```python
from build123d import *

# Parameters (mm, degrees)
Y_KSEKLIK_EKSTR_ZYON1_DEPTH = 12
Y_KSEKLIK_EKSTR_ZYON2_DEPTH = 6
IZIM1_4_R                   = 19
IZIM1_4_R_2                 = 12
Y_KSEKLIK_EKSTR_ZYON3_DEPTH = 12
IZIM1_5_W                   = 6
IZIM1_5_H                   = 10
Y_KSEKLIK_EKSTR_ZYON4_DEPTH = 6
KES_EKSTR_ZYON1_DEPTH       = 11
F_6_0_6_AP_DELIK1_D         = 6
KES_EKSTR_ZYON2_DEPTH       = 4
RADYUS1_R                   = 1
RADYUS2_R                   = 1
IZIM9_R                     = 1
KES_EKSTR_ZYON3_DEPTH       = 50
IZIM10_R                    = 1
KES_EKSTR_ZYON4_DEPTH       = 16
RADYUS3_R                   = 2


with BuildPart() as part:
    # Çizim1 → Yükseklik-Ekstrüzyon1 (new body, symmetric)
    with BuildSketch(Plane.XY):
        with BuildLine():
            Line((-20, 0), (-15, 0))
            ThreePointArc((-15, 0), (0, 15), (15, 0))
            Line((15, 0), (20, 0))
            ThreePointArc((20, 0), (0, 20), (-20, 0))
        make_face()
    extrude(amount=Y_KSEKLIK_EKSTR_ZYON1_DEPTH, both=True)

    # Çizim1<3> → Yükseklik-Ekstrüzyon2 (add, symmetric)
    with BuildSketch(Plane.XY):
        with BuildLine():
            Line((-10, 82.394505579), (-16.180060624, 11.756089409))
            ThreePointArc((-16.180060624, 11.756089409), (0, 20), (16.180060624, 11.756089409))
            Line((16.180060624, 11.756089409), (10, 82.394505579))
            ThreePointArc((10, 82.394505579), (0, 79.55), (-10, 82.394505579))
        make_face()
    extrude(amount=Y_KSEKLIK_EKSTR_ZYON2_DEPTH, both=True)

    # Çizim1<4> → Yükseklik-Ekstrüzyon3 (add, symmetric)
    with BuildSketch(Plane.XY):
        with Locations((0, 98.55)):
            Circle(IZIM1_4_R)
        with Locations((0, 98.55)):
            Circle(IZIM1_4_R_2, mode=Mode.SUBTRACT)
    extrude(amount=Y_KSEKLIK_EKSTR_ZYON3_DEPTH, both=True)

    # Çizim1<5> → Yükseklik-Ekstrüzyon4 (add, symmetric)
    with BuildSketch(Plane.XY):
        with Locations((-27, 5)):
            Rectangle(IZIM1_5_W, IZIM1_5_H)
        with BuildLine():
            Line((-24, 0), (-20, 0))
            ThreePointArc((-20, 0), (-19.318516526, 5.176380902), (-17.320508076, 10))
            Line((-17.320508076, 10), (-24, 10))
            Line((-24, 10), (-24, 0))
        make_face()
        with BuildLine():
            ThreePointArc((17.320508076, 10), (19.318516526, 5.176380902), (20, 0))
            Line((20, 0), (24, 0))
            Line((24, 0), (24, 10))
            Line((24, 10), (17.320508076, 10))
        make_face()
        with Locations((27, 5)):
            Rectangle(IZIM1_5_W, IZIM1_5_H)
    extrude(amount=Y_KSEKLIK_EKSTR_ZYON4_DEPTH, both=True)

    # Çizim2 → Kes-Ekstrüzyon1 (cut, through all)
    with BuildSketch(Plane(origin=(0, 10, 0), x_dir=(1, 0, 0), z_dir=(0, 1, 0))):
        with BuildLine():
            ThreePointArc((-30, 0), (-28.242640687, 4.242640687), (-24, 6))
            Line((-24, 6), (-30, 6))
            Line((-30, 6), (-30, 0))
        make_face()
        with BuildLine():
            Line((-30, -6), (-24, -6))
            ThreePointArc((-24, -6), (-28.242640687, -4.242640687), (-30, 0))
            Line((-30, 0), (-30, -6))
        make_face()
    kes_ekstr_zyon1 = extrude(amount=-KES_EKSTR_ZYON1_DEPTH, mode=Mode.SUBTRACT)

    # Ø6.0 (6) Çap Delik1 (through all)
    with Locations(Plane(origin=(0, 10, 0), x_dir=(1, 0, 0), z_dir=(0, 1, 0))):
        with Locations((-24, 0)):
            f_6_0_6_ap_delik1 = Hole(F_6_0_6_AP_DELIK1_D / 2)

    # Aynalama1: Ø6.0 (6) Çap Delik1 across plane
    add(f_6_0_6_ap_delik1.mirror(Plane(origin=(0, 0, 0), x_dir=(0, 0, 1), z_dir=(1, 0, 0))), mode=Mode.SUBTRACT)

    # Çizim8 → Kes-Ekstrüzyon2 (cut)
    with BuildSketch(Plane.XY.offset(6)):
        with BuildLine():
            Line((5.845451143, 72.512650075), (9.562487885, 30.026725708))
            ThreePointArc((9.562487885, 30.026725708), (9.044653162, 28.501233808), (7.570098489, 27.852414223))
            Line((7.570098489, 27.852414223), (-7.570098489, 27.852414223))
            ThreePointArc((-7.570098489, 27.852414223), (-9.044653162, 28.501233808), (-9.562487885, 30.026725708))
            Line((-9.562487885, 30.026725708), (-5.845451143, 72.512650075))
            ThreePointArc((-5.845451143, 72.512650075), (-5.204242163, 73.812893263), (-3.853061747, 74.338338589))
            Line((-3.853061747, 74.338338589), (3.853061747, 74.338338589))
            ThreePointArc((3.853061747, 74.338338589), (5.204242163, 73.812893263), (5.845451143, 72.512650075))
        make_face()
    kes_ekstr_zyon2 = extrude(amount=-KES_EKSTR_ZYON2_DEPTH, mode=Mode.SUBTRACT)

    # Aynalama2: Kes-Ekstrüzyon2 across plane
    add(kes_ekstr_zyon2.mirror(Plane.XY), mode=Mode.SUBTRACT)

    # Radyus1
    radyus1_edges = [part.edges().sort_by_distance(p)[0] for p in [
        (5.204242163, 73.812893263, 2),
        (7.703969514, 51.269687892, 2),
        (9.044653162, 28.501233808, 2),
        (0, 27.852414223, 2),
        (-9.044653162, 28.501233808, 2),
        (-7.703969514, 51.269687892, 2),
        (-5.204242163, 73.812893263, 2),
        (0, 74.338338589, 2),
        (5.204242163, 73.812893263, 6),
        (0, 74.338338589, 6),
        (-5.204242163, 73.812893263, 6),
        (-7.703969514, 51.269687892, 6),
        (-9.044653162, 28.501233808, 6),
        (0, 27.852414223, 6),
        (9.044653162, 28.501233808, 6),
        (7.703969514, 51.269687892, 6),
    ]]
    fillet(radyus1_edges, radius=RADYUS1_R)

    # Radyus2
    radyus2_edges = [part.edges().sort_by_distance(p)[0] for p in [
        (5.204242163, 73.812893263, -6),
        (0, 74.338338589, -6),
        (-5.204242163, 73.812893263, -6),
        (-7.703969514, 51.269687892, -6),
        (-9.044653162, 28.501233808, -6),
        (0, 27.852414223, -6),
        (9.044653162, 28.501233808, -6),
        (7.703969514, 51.269687892, -6),
        (5.204242163, 73.812893263, -2),
        (0, 74.338338589, -2),
        (-5.204242163, 73.812893263, -2),
        (-7.703969514, 51.269687892, -2),
        (-9.044653162, 28.501233808, -2),
        (0, 27.852414223, -2),
        (9.044653162, 28.501233808, -2),
        (7.703969514, 51.269687892, -2),
    ]]
    fillet(radyus2_edges, radius=RADYUS2_R)

    # Aynalama3: Kes-Ekstrüzyon1 across plane
    add(kes_ekstr_zyon1.mirror(Plane(origin=(0, 0, 0), x_dir=(0, 0, 1), z_dir=(1, 0, 0))), mode=Mode.SUBTRACT)

    # Çizim9 → Kes-Ekstrüzyon3 (cut, through all)
    with BuildSketch(Plane(origin=(19, 0, 0), x_dir=(0, 0, -1), z_dir=(1, 0, 0))):
        with Locations((0, 98.55)):
            Circle(IZIM9_R)
    extrude(amount=-KES_EKSTR_ZYON3_DEPTH, mode=Mode.SUBTRACT)

    # Çizim10 → Kes-Ekstrüzyon4 (cut)
    with BuildSketch(Plane(origin=(0, 117.55, 0), x_dir=(1, 0, 0), z_dir=(0, 1, 0))):
        Circle(IZIM10_R)
    extrude(amount=-KES_EKSTR_ZYON4_DEPTH, mode=Mode.SUBTRACT)

    # Radyus3
    radyus3_edges = [part.edges().sort_by_distance(p)[0] for p in [
        (10, 82.394505579, 0),
        (-10, 82.394505579, 0),
    ]]
    fillet(radyus3_edges, radius=RADYUS3_R)


solid = part.part
```
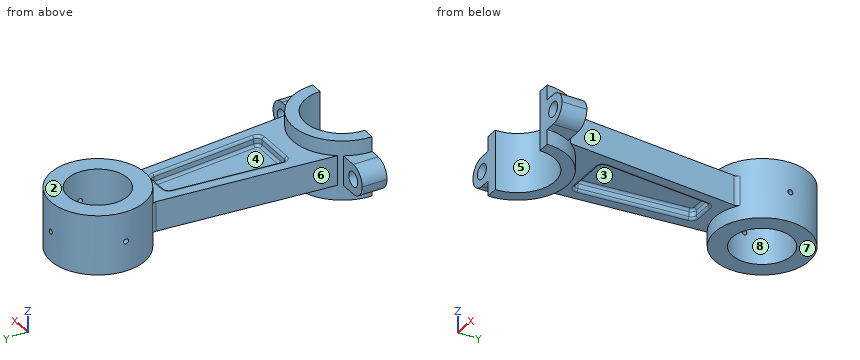
Check sheet for the modelled part. Datum: model origin and axes. Units: mm. Face numbers are marked on the shaded views. A direction names the side the tool comes from. Give positions to 0.01 mm unless a question says otherwise; leave off trailing zeros. Write each loop counter-clockwise with the first axis right and the second up, starting at its lowest first coordinate (ties: lowest second). Pieces come first, ordered by that corner, then holes. Notation, with made-up numbers: (71, -7.5) -> (96, -7.5) arc R21 ccw to (96, 24.5) -> close; hole circle Ø5 at (82, 23). An arc over 180 degrees is marked (long way). Use CSV: the item, a comma, the result in double quotes. Start each with the question number.
Q1. Cross-section at A-A on z = 8. Enter the section's corners in (x, y), and give its area (3 significant figures).
Q2. Scan lines: line 1 along Y through (x, z) = (0, -4.5); line 2 along Y through (x, z) = (-10.5, 10.75); line 3 along X through (y, z) = (88, 1.75). Record each from-to range of solid material in increasing order.
Q3. Depth check by flat-ended pin: P1, Ø3, axis at y = 98.55, z = 0, coming from the -X side; P2, Ø1.6, axis at x = -1, z = 4.5, coming from the -Y side; P3, Ø12, axis at y = 22, z = -1, coming from the +X side; P4, Ø5.5, axis at x = -24, z = 0, coming from the +Y side. Enter the tip coordinate at first touch or a pass-through.
Q4. Cross-section at C-C on x = -25.5. Enter the section's corners in (y, z), and give its area (3 significant figures).
Q5. Tool access check on the marked faces 1, 2, 3 and 4. Record the directions out of +Z, -Z, +X, -X, +Y, -Y that give a thin tool (end or side, any length) a straight path to the whole face; none if there is none.
Q6. Release check for a two-part mould opening along X. For the marked faces 5, 6, 7 and 8 record: +X half, -X half, draft (parallel to the pull), parting line (faces both ways), or undercut.
Working result:
1,outline,"(-20, 0) -> (-15, 0) arc R15 cw to (15, 0) -> (20, 0) arc R20 ccw to start; circle Ø38 at (0, 98.55); hole circle Ø24 at (0, 98.55)"
1,area,"957 mm^2"
2,line 1,"y = 15 to 27.85, 74.34 to 86.55, 110.55 to 117.55"
2,line 2,"y = 10.71 to 17.02, 82.71 to 92.74, 104.36 to 114.39"
2,line 3,"x = -15.8 to -5.72, 5.72 to 15.8"
3,P1,"stops at x = -19"
3,P2,"stops at y = 14.89"
3,P3,"stops at x = 15.81"
3,P4,"passes through"
4,outline,"(0, -5.81) -> (10, -5.81) -> (10, -2.6) -> (0, -2.6) -> close; (0, 2.6) -> (10, 2.6) -> (10, 5.81) -> (0, 5.81) -> close"
4,area,"64.2 mm^2"
5,face 1,"+Z, -Z, +X"
5,face 2,"+Z, +X, -X, +Y, -Y"
5,face 3,"-Z"
5,face 4,"+Z"
6,face 5,"undercut"
6,face 6,"-X half"
6,face 7,"draft"
6,face 8,"undercut"
